Check sheet for the modelled part. Datum: model origin and axes. Units: mm. A direction names the side the tool comes from. Round coordinates to 2 decimals unless told otherwise and drop trailing zeros. Loops run counter-clockwise (first coordinate to the right, second up) from the corner with the lowest first, then second, coordinate; pieces in that order, holes last. Notation, with made-up numbers: (-21.5, 82) - (28.5, 82) arc R26 ccw to (28.5, 104) - close; hole circle Ø10 at (69.25, 77). An arc over 180 degrees is marked (long way). Put each result on its own line as item: value.
```python
from build123d import *

# Parameters (mm, degrees)
SKETCH_W          = 124.4
SKETCH_H          = 132
PAD_DEPTH         = 4
SKETCH001_W       = 4
SKETCH001_H       = 132
PAD001_DEPTH      = 19.6
PAD002_DEPTH      = 132
SKETCH003_W       = 10.5
SKETCH003_H       = 4.25
POCKET_DEPTH      = 4.001
POCKET_DEPTH_BACK = 21.601
FILLET_R          = 6
FILLET001_R       = 2
FILLET002_R       = 1
SKETCH004_W       = 47
SKETCH004_H       = 3
PAD003_DEPTH      = 14
SKETCH005_R       = 1.55
SKETCH005_W       = 40
SKETCH005_H       = 10
POCKET001_DEPTH   = 4.001
SKETCH006_W       = 52
SKETCH006_H       = 10
POCKET002_DEPTH   = 2
SKETCH007_W       = 12.5
SKETCH007_H       = 11
POCKET003_DEPTH   = 4.001
SKETCH008_W       = 7
SKETCH008_H       = 4.5
SKETCH008_W_2     = 10
PAD004_DEPTH      = 15
SKETCH009_W       = 7
SKETCH009_H       = 1.5
SKETCH009_W_2     = 10
POCKET004_DEPTH   = 21.601
SKETCH010_R       = 1.65
POCKET005_DEPTH   = 132.001
POCKET006_DEPTH   = 4.001
CHAMFER_SIZE      = 3
CHAMFER001_SIZE   = 2


with BuildPart() as part:
    # Sketch → Pad (new body)
    with BuildSketch(Plane.XY):
        with Locations((0, 66)):
            Rectangle(SKETCH_W, SKETCH_H)
    extrude(amount=-PAD_DEPTH)

    # Sketch001 → Pad001 (join)
    with BuildSketch(Plane.XY):
        with Locations((-60.2, 66)):
            Rectangle(SKETCH001_W, SKETCH001_H)
        with Locations((60.2, 66)):
            Rectangle(SKETCH001_W, SKETCH001_H)
    extrude(amount=PAD001_DEPTH)

    # Sketch002 → Pad002 (join)
    with BuildSketch(Plane.XZ):
        Polygon((-58.2, 19.6), (-62.2, 19.6), (-60.2, 21.6), align=None)
        Polygon((58.2, 19.6), (62.2, 19.6), (60.2, 21.6), align=None)
    extrude(amount=-PAD002_DEPTH)

    # Sketch003 → Pocket (cut, two sides)
    with BuildSketch(Plane.XY) as pocket_sk:
        with Locations((-35, 6.125)):
            Rectangle(SKETCH003_W, SKETCH003_H)
        with Locations((-35, 66.125)):
            Rectangle(SKETCH003_W, SKETCH003_H)
        with Locations((-35, 129.875)):
            Rectangle(SKETCH003_W, SKETCH003_H)
        with Locations((35, 6.125)):
            Rectangle(SKETCH003_W, SKETCH003_H)
        with Locations((35, 66.125)):
            Rectangle(SKETCH003_W, SKETCH003_H)
        with Locations((35, 129.875)):
            Rectangle(SKETCH003_W, SKETCH003_H)
        Polygon((-42.75, 0), (-27.25, 0), (-22.25, 4), (22.25, 4), (27.25, 0), (42.75, 0), (47.75, 4), (90, 4), (90, -46), (-90, -46), (-90, 4), (-47.75, 4), align=None)
    extrude(amount=-POCKET_DEPTH, mode=Mode.SUBTRACT)
    extrude(pocket_sk.sketch, amount=POCKET_DEPTH_BACK, mode=Mode.SUBTRACT)

    # Fillet
    fillet_edges = [part.edges().sort_by_distance(p)[0] for p in [
        (-62.2, 68, -4),
        (62.2, 68, -4),
    ]]
    fillet(fillet_edges, radius=FILLET_R)

    # Fillet001
    fillet001_edges = [part.edges().sort_by_distance(p)[0] for p in [
        (-58.2, 68, 0),
        (58.2, 68, 0),
    ]]
    fillet(fillet001_edges, radius=FILLET001_R)

    # Fillet002
    fillet002_edges = [part.edges().sort_by_distance(p)[0] for p in [
        (-40.25, 129.875, 0),
        (-29.75, 129.875, 0),
        (29.75, 129.875, 0),
        (40.25, 129.875, 0),
        (29.75, 66.125, 0),
        (40.25, 66.125, 0),
        (29.75, 6.125, 0),
        (40.25, 6.125, 0),
        (-40.25, 6.125, 0),
        (-29.75, 6.125, 0),
        (-40.25, 66.125, 0),
        (-29.75, 66.125, 0),
    ]]
    fillet(fillet002_edges, radius=FILLET002_R)

    # Sketch004 → Pad003 (new body)
    with BuildSketch(Plane.XY):
        with Locations((-34.7, 96.5)):
            Rectangle(SKETCH004_W, SKETCH004_H)
    extrude(amount=PAD003_DEPTH)

    # Sketch005 → Pocket001 (cut, through all)
    with BuildSketch(Plane.XY):
        with Locations((7, 55)):
            Circle(SKETCH005_R)
        with Locations((53, 55)):
            Circle(SKETCH005_R)
        with Locations((30, 55)):
            Rectangle(SKETCH005_W, SKETCH005_H)
    extrude(amount=-POCKET001_DEPTH, mode=Mode.SUBTRACT)

    # Sketch006 (on DatumPlane) → Pocket002 (cut)
    with BuildSketch(Plane.XY.offset(-4)):
        with Locations((30, 55)):
            Rectangle(SKETCH006_W, SKETCH006_H)
    extrude(amount=POCKET002_DEPTH, mode=Mode.SUBTRACT)

    # Sketch007 → Pocket003 (cut, through all)
    with BuildSketch(Plane.XY):
        with Locations((42.25, 115.5)):
            Rectangle(SKETCH007_W, SKETCH007_H)
    extrude(amount=-POCKET003_DEPTH, mode=Mode.SUBTRACT)

    # Sketch008 → Pad004 (join)
    with BuildSketch(Plane.XY):
        with Locations((52, 109.25)):
            Rectangle(SKETCH008_W, SKETCH008_H)
        with Locations((31, 109.25)):
            Rectangle(SKETCH008_W_2, SKETCH008_H)
    extrude(amount=PAD004_DEPTH)

    # Sketch009 → Pocket004 (cut, through all)
    with BuildSketch(Plane.XY):
        with Locations((52, 109.25)):
            Rectangle(SKETCH009_W, SKETCH009_H)
        with Locations((31, 109.25)):
            Rectangle(SKETCH009_W_2, SKETCH009_H)
    extrude(amount=POCKET004_DEPTH, mode=Mode.SUBTRACT)

    # Sketch010 → Pocket005 (cut, through all)
    with BuildSketch(Plane.XZ):
        with Locations((32, 11.65)):
            Circle(SKETCH010_R)
        with Locations((52, 11.65)):
            Circle(SKETCH010_R)
    extrude(amount=-POCKET005_DEPTH, mode=Mode.SUBTRACT)

    # Sketch011 → Pocket006 (cut, through all)
    with BuildSketch(Plane.XY):
        with BuildLine():
            ThreePointArc((5, 103), (4, 104), (3, 103))
            Line((3, 103), (3, 73))
            ThreePointArc((3, 73), (4, 72), (5, 73))
            Line((5, 103), (5, 73))
        make_face()
        with BuildLine():
            ThreePointArc((11, 103), (10, 104), (9, 103))
            Line((9, 103), (9, 73))
            ThreePointArc((9, 73), (10, 72), (11, 73))
            Line((11, 103), (11, 73))
        make_face()
        with BuildLine():
            ThreePointArc((17, 103), (16, 104), (15, 103))
            Line((15, 103), (15, 73))
            ThreePointArc((15, 73), (16, 72), (17, 73))
            Line((17, 103), (17, 73))
        make_face()
        with BuildLine():
            ThreePointArc((23, 103), (22, 104), (21, 103))
            Line((21, 103), (21, 73))
            ThreePointArc((21, 73), (22, 72), (23, 73))
            Line((23, 103), (23, 73))
        make_face()
        with BuildLine():
            ThreePointArc((29, 103), (28, 104), (27, 103))
            Line((27, 103), (27, 73))
            ThreePointArc((27, 73), (28, 72), (29, 73))
            Line((29, 103), (29, 73))
        make_face()
        with BuildLine():
            ThreePointArc((35, 103), (34, 104), (33, 103))
            Line((33, 103), (33, 73))
            ThreePointArc((33, 73), (34, 72), (35, 73))
            Line((35, 103), (35, 73))
        make_face()
        with BuildLine():
            ThreePointArc((41, 103), (40, 104), (39, 103))
            Line((39, 103), (39, 73))
            ThreePointArc((39, 73), (40, 72), (41, 73))
            Line((41, 103), (41, 73))
        make_face()
        with BuildLine():
            ThreePointArc((47, 103), (46, 104), (45, 103))
            Line((45, 103), (45, 73))
            ThreePointArc((45, 73), (46, 72), (47, 73))
            Line((47, 103), (47, 73))
        make_face()
        with BuildLine():
            ThreePointArc((53, 103), (52, 104), (51, 103))
            Line((51, 103), (51, 73))
            ThreePointArc((51, 73), (52, 72), (53, 73))
            Line((53, 103), (53, 73))
        make_face()
    extrude(amount=-POCKET006_DEPTH, mode=Mode.SUBTRACT)

    # Chamfer
    chamfer_edges = [part.edges().sort_by_distance(p)[0] for p in [
        (31, 111.5, 0),
        (52, 111.5, 0),
    ]]
    chamfer(chamfer_edges, length=CHAMFER_SIZE)

    # Chamfer001
    chamfer001_edges = [part.edges().sort_by_distance(p)[0] for p in [
        (31, 107, 0),
        (52, 107, 0),
    ]]
    chamfer(chamfer001_edges, length=CHAMFER001_SIZE)


solid = part.part
```
Item 1: Section check A-A on x = 12.5. Enter the section's corners in (y, z).
Filled sheet:
outline: (4, -4) - (50, -4) - (50, 0) - (4, 0) - close; (60, -4) - (132, -4) - (132, 0) - (60, 0) - close
Item 2: Release check for a two-part mould opening along Z. For faces 6 (the flat face through (52, 110, 7)), 7 (the flat face through (52, 113, 1.5)), 8 (the cylindrical face through (30.35, 107.74, 11.72)) record: +Z half, -Z half, draft (parallel to the pull), parting line (faces both ways), or undercut.
Filled sheet:
face 6: draft
face 7: +Z half
face 8: undercut
Item 3: Tool access check on faces 1 (the flat face through (31, 108.5, 7)), 2 (the flat face through (51, 88, -2)), 3 (the flat face through (31, 107, 8)), 4 (the flat face through (-40.25, 130, -2)), 5 (the flat face through (55.5, 111, 6)). Record the directions out of +Z, -Z, +X, -X, +Y, -Y that give a thin tool (end or side, any length) a straight path to the whole face; none if there is none.
Filled sheet:
face 1: +Z
face 2: +Z, -Z
face 3: +Z, -Y
face 4: +Z, -Z, +Y
face 5: +Z, +Y, -Y
Item 4: Section check B-B on z = 5.25. Enter the section's corners in (x, y).
Filled sheet:
outline: (-62.2, 4) - (-58.2, 4) - (-58.2, 95) - (-11.2, 95) - (-11.2, 98) - (-58.2, 98) - (-58.2, 132) - (-62.2, 132) - close; (26, 107) - (36, 107) - (36, 108.5) - (26, 108.5) - close; (26, 110) - (36, 110) - (36, 111.5) - (26, 111.5) - close; (48.5, 107) - (55.5, 107) - (55.5, 108.5) - (48.5, 108.5) - close; (48.5, 110) - (55.5, 110) - (55.5, 111.5) - (48.5, 111.5) - close; (58.2, 4) - (62.2, 4) - (62.2, 132) - (58.2, 132) - close
Item 5: Thickness scan on line 1 (Y direction, x = 8, z = -2.25); line 2 (Z direction, x = 52, y = 107.55); line 3 (X direction, y = 64, z = 16.5). Record the ranges inside material, lowest first. Write a range as from..to.
Filled sheet:
line 1: 4..50, 60..132
line 2: -4..10, 13.3..15
line 3: -62.2..-58.2, 58.2..62.2
Item 6: Go/stop test with flat-tipped pins: pin 1 (11 mm diameter, centred on x = -39, z = 6, fed in from +Y); pin 2 (1.2 mm diameter, centred on y = 90, z = -2.5, fed in from -X); pin 3 (2 mm diameter, centred on y = 91.5, z = -2.5, fed in from +X). Record where each tip stops, or that it passes through.
Filled sheet:
pin 1: y = 98
pin 2: x = -60.76
pin 3: x = 61.07
Item 7: Section check C-C on x = -32.5. Enter the section's corners in (y, z).
Filled sheet:
outline: (0, -4) - (4, -4) - (4, 0) - (0, 0) - close; (8.25, -4) - (64, -4) - (64, 0) - (8.25, 0) - close; (68.25, -4) - (127.75, -4) - (127.75, 0) - (98, 0) - (98, 14) - (95, 14) - (95, 0) - (68.25, 0) - close
Item 8: Section check D-D on y = 43.5. Enter the section's corners in (x, z), then the cut area to 3 significant figures.
Filled sheet:
outline: (-62.2, 2) arc R6 ccw to (-56.2, -4) - (56.2, -4) arc R6 ccw to (62.2, 2) - (62.2, 19.6) - (60.2, 21.6) - (58.2, 19.6) - (58.2, 2) arc R2 cw to (56.2, 0) - (-56.2, 0) arc R2 cw to (-58.2, 2) - (-58.2, 19.6) - (-60.2, 21.6) - (-62.2, 19.6) - close
area: 649 mm²
